Autodesk Inventor part; units mm, degrees
ref_plane "YZ Plane" through (0, 0, 0) normal (1, 0, 0) x (0, 1, 0)
ref_plane "XZ Plane" through (0, 0, 0) normal (0, 1, 0) x (-1, 0, 0)
ref_plane "XY Plane" through (0, 0, 0) normal (0, 0, 1) x (1, 0, 0)
sketch "Sketch1" plane through (0, 0, 0) normal (0, 1, 0) x (-1, 0, 0)
  line L0 (0, 0) -> (17.3205, 0)
  line L1 (0, -262) -> (0, 0)
  line L2 (17.3205, -272) -> (0, -262)
  line L3 (17.3205, -108) -> (8.3205, -108)
  line L4 (8.3205, -108) -> (8.3205, -120)
  line L5 (8.3205, -120) -> (17.3205, -120)
  line L6 (17.3205, 0) -> (17.3205, -108)
  line L7 (17.3205, -120) -> (17.3205, -272)
  dimension "d0" = 272
  dimension "d1" = 60
  dimension "d2" = 12
  dimension "d3" = 9
  dimension "d4" = 108
  dimension "d6" = 262
extrude "Extrusion1" add sketch "Sketch1" along normal mid plane 6
sketch "Sketch2" plane through (0, 3, 0) normal (0, 1, 0) x (1, 0, 0)
  line L0 (0, 0) -> (0, 262)
  point P0 (-10, 13)
  point P1 (-10, 42)
  point P2 (-10, 71)
  point P3 (-10, 100)
  point P4 (-10, 129)
  point P5 (-10, 158)
  point P6 (-10, 187)
  point P7 (-10, 216)
  point P8 (-10, 245)
  dimension "d9" = 10
  dimension "d10" = 17
  dimension "d11" = 13
  dimension "d12" = 29
  dimension "d13" = 29
  dimension "d14" = 29
  dimension "d15" = 29
  dimension "d16" = 29
  dimension "d17" = 29
  dimension "d18" = 29
  dimension "d19" = 29
hole "Hole1" at (-10, 3, -13) at (-10, 3, -42) at (-10, 3, -71) at (-10, 3, -100) at (-10, 3, -129) at (-10, 3, -158) at (-10, 3, -187) at (-10, 3, -216) at (-10, 3, -245) direction (0, -1, 0) diameter 5 depth 6
sketch "Sketch3" plane through (0, 3, 0) normal (0, 1, 0) x (1, 0, 0)
  line L0 (0, 0) -> (-17.3205, 0)
  line L1 (0, 262) -> (0, 0)
  line L2 (-5, 0) -> (0, 0)
  line L3 (0, 0) -> (0, 262)
  line L4 (0, 262) -> (-5, 262)
  line L5 (-5, 262) -> (-5, 0)
  dimension "d27" = 5
extrude "Extrusion2" add sketch "Sketch3" along normal blind 13
sketch "Sketch4" plane through (-5, 3, -262) normal (-1, 0, 0) x (0, 0, 1)
  line L0 (0, 13) -> (262, 13)
  line L1 (154, 13) -> (154, 7)
  line L2 (154, 7) -> (142, 7)
  line L3 (142, 7) -> (142, 13)
  line L4 (262, 0) -> (262, 13)
  point P0 (262, -3)
  dimension "d30" = 12
  dimension "d31" = 6
  dimension "d32" = 108
extrude "Extrusion3" cut sketch "Sketch4" against normal blind 5
sketch "Sketch5" plane through (-5, 3, -262) normal (-1, 0, 0) x (0, 0, 1)
  line L0 (262, 0) -> (262, 13)
  line L1 (154, 13) -> (154, 7)
  line L2 (262, -6) -> (154, -6)
  point P0 (262, -3)
  point P1 (256, 4)
  point P2 (227, 4)
  point P3 (198, 4)
  point P4 (169, 4)
  point P5 (262, 6.5)
  dimension "d35" = 6
  dimension "d36" = 15
  dimension "d37" = 29
  dimension "d38" = 29
  dimension "d39" = 29
  dimension "d40" = 10
hole "Hole2" at (-5, 7, -6) at (-5, 7, -35) at (-5, 7, -64) at (-5, 7, -93) direction (1, 0, 0) diameter 4 depth 5 countersink diameter 5 countersink angle 90
sketch "Sketch6" plane through (-5, 3, -262) normal (-1, 0, 0) x (0, 0, 1)
  circle A0 centre (169, 4) radius 2.5
  circle A1 centre (198, 4) radius 2.5
  circle A2 centre (227, 4) radius 2.5
  circle A3 centre (256, 4) radius 2.5
  line L0 (154, 13) -> (154, 7)
  line L1 (154, 7) -> (142, 7)
  line L2 (142, 7) -> (142, 13)
  line L3 (0, 13) -> (142, 13)
  line L4 (0, 0) -> (0, 13)
  line L5 (262, 0) -> (0, 0)
  line L6 (262, 0) -> (262, 13)
  line L7 (154, 13) -> (262, 13)
  line L8 (0, 0) -> (46, 13)
  point P0 (262, -3)
  dimension "d48" = 96
extrude "Extrusion4" cut sketch "Sketch6" against normal up to surface (5 mm away) contours L4 L3 L8
fillet "Fillet1" radius 2 1 edges at (-17.3205, 0, -272)
properties part number "1013"
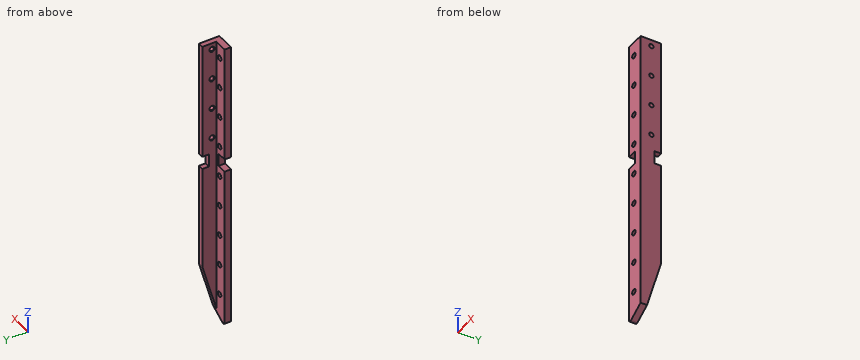
Verification items for the finished model (mm, model axes). Round coordinates to 2 decimals unless told otherwise and drop trailing zeros. Loops run counter-clockwise (first coordinate to the right, second up) from the corner with the lowest first, then second, coordinate; pieces in that order, holes last. Notation, with made-up numbers: (10.5, 55) - (37.5, 55) arc R24 ccw to (37.5, 88) - close; hole circle Ø5 at (33.25, 75). An arc over 180 degrees is marked (long way). Write item = value, one per line.
Q1. Depth check by flat-ended pin: pin 1 (3 mm diameter, centred on x = -10, z = -187, fed in from -Y); pin 2 (1.8 mm diameter, centred on y = 0.5, z = -115, fed in from -X); pin 3 (6.5 mm diameter, centred on y = 7, z = -64, fed in from -X); pin 4 (6 mm diameter, centred on x = -10, z = -13, fed in from +Y). Enter the tip coordinate at first touch or a pass-through.
Here are the results:
pin_1 = through
pin_2 = -8.32
pin_3 = -5
pin_4 = 3
Q2. Sectioned sample at C-C on z = -251.5. Record the boundary of the cut face in (x, y), plus the area to 3 significant figures.
Here are the results:
outline = (-17.32, -3) - (0, -3) - (0, 5.97) - (-5, 5.97) - (-5, 3) - (-17.32, 3) - close
area = 119 mm^2
Q3. Material ranges on L1, parallel to Y at x = -2.4, z = -35; L2, parallel to X at y = 0.6, z = -187; L3, parallel to X at y = 7.25, z = -162, recorded low to high.
Here are the results:
L1 = -3 to 5, 9 to 16
L2 = -17.32 to -12.5, -7.5 to 0
L3 = -5 to 0
Q4. Sectioned sample at A-A on z = -158. Record the boundary of the cut face in (x, y).
Here are the results:
outline = (-17.32, -3) - (-12.5, -3) - (-12.5, 3) - (-17.32, 3) - close; (-7.5, -3) - (0, -3) - (0, 16) - (-5, 16) - (-5, 3) - (-7.5, 3) - close
Q5. Sectioned sample at B-B on y = 0. State how many separate pieces and enclosed holes the cut face has, plus the area to 3 significant figures.
Here are the results:
separate_pieces = 1
enclosed_holes = 9
area = 4,340 mm^2
